```python
from build123d import *

# Parameters (mm, degrees)
SKETCH1_W           = 304.8
SKETCH1_H           = 101.6
BOSS_EXTRUDE1_DEPTH = 6.35
SKETCH2_R           = 12.7
BOSS_EXTRUDE3_DEPTH = 5.55625
SKETCH9_R           = 11.1125
CUT_EXTRUDE4_DEPTH  = 4.445
CUT_EXTRUDE5_START  = -5.55625
SKETCH10_R          = 11.1125
CUT_EXTRUDE5_DEPTH  = 5.55625
SKETCH11_R          = 7.9375
CUT_EXTRUDE6_DEPTH  = 310.094403462
SKETCH12_R          = 12.7
CUT_EXTRUDE7_DEPTH  = 310.0695755
SKETCH22_W          = 63.5
SKETCH22_H          = 63.5
BOSS_EXTRUDE7_DEPTH = 12.7
SKETCH25_W          = 50.8
SKETCH25_H          = 50.8
CUT_EXTRUDE11_DEPTH = 15.24
SKETCH18_W          = 40.386
SKETCH18_H          = 20.066
BOSS_EXTRUDE5_DEPTH = 39.878
SKETCH32_R          = 4.7625
CUT_EXTRUDE12_DEPTH = 6.35


with BuildPart() as part:
    # Sketch1 → Boss-Extrude1 (new body)
    with BuildSketch(Plane(origin=(0, 0, 0), x_dir=(1, 0, 0), z_dir=(0, 1, 0))):
        with Locations((-152.4, 0)):
            Rectangle(SKETCH1_W, SKETCH1_H)
    extrude(amount=BOSS_EXTRUDE1_DEPTH)

    # Sketch2 → Boss-Extrude3 (add)
    with BuildSketch(Plane(origin=(0, 6.35, 0), x_dir=(1, 0, 0), z_dir=(0, 1, 0))):
        with Locations(Location((-282.839226834, 0, 0), (0, 0, 90))):
            Circle(SKETCH2_R)
    extrude(amount=BOSS_EXTRUDE3_DEPTH)

    # Sketch9 → Cut-Extrude4 (cut)
    with BuildSketch(Plane(origin=(0, 11.90625, 0), x_dir=(1, 0, 0), z_dir=(0, 1, 0))):
        with Locations(Location((-282.839226834, 0, 0), (0, 0, 270))):
            Circle(SKETCH9_R)
    extrude(amount=-CUT_EXTRUDE4_DEPTH, mode=Mode.SUBTRACT)

    # Sketch10 → Cut-Extrude5 (cut)
    with BuildSketch(Plane(origin=(0, 0, 0), x_dir=(-1, 0, 0), z_dir=(0, -1, 0)).offset(CUT_EXTRUDE5_START)):
        with Locations(Location((282.839226834, 0, 0), (0, 0, 270))):
            Circle(SKETCH10_R)
    extrude(amount=CUT_EXTRUDE5_DEPTH, mode=Mode.SUBTRACT)

    # Sketch11 → Cut-Extrude6 (cut, through all)
    with BuildSketch(Plane(origin=(0, 7.46125, 0), x_dir=(1, 0, 0), z_dir=(0, 1, 0))):
        with Locations(Location((-282.839226834, 0, 0), (0, 0, 270))):
            Circle(SKETCH11_R)
    extrude(amount=-CUT_EXTRUDE6_DEPTH, mode=Mode.SUBTRACT)

    # Sketch12 → Cut-Extrude7 (cut, through all)
    with BuildSketch(Plane(origin=(0, 6.35, 0), x_dir=(1, 0, 0), z_dir=(0, 1, 0))):
        with Locations(Location((-134.666203771, 0, 0), (0, 0, 270))):
            Circle(SKETCH12_R)
    extrude(amount=-CUT_EXTRUDE7_DEPTH, mode=Mode.SUBTRACT)

    # Sketch22 → Boss-Extrude7 (add)
    with BuildSketch(Plane(origin=(0, 6.35, 0), x_dir=(1, 0, 0), z_dir=(0, 1, 0))):
        with Locations((-134.666203771, 0)):
            Rectangle(SKETCH22_W, SKETCH22_H)
    extrude(amount=BOSS_EXTRUDE7_DEPTH)

    # Sketch25 → Cut-Extrude11 (cut)
    with BuildSketch(Plane(origin=(0, 19.05, 0), x_dir=(1, 0, 0), z_dir=(0, 1, 0))):
        with Locations((-134.666203771, 0)):
            Rectangle(SKETCH25_W, SKETCH25_H)
    extrude(amount=-CUT_EXTRUDE11_DEPTH, mode=Mode.SUBTRACT)

    # Sketch18 → Boss-Extrude5 (add)
    with BuildSketch(Plane(origin=(0, 6.35, 0), x_dir=(1, 0, 0), z_dir=(0, 1, 0))):
        with Locations((-206.419013169, 0)):
            Rectangle(SKETCH18_W, SKETCH18_H)
    extrude(amount=BOSS_EXTRUDE5_DEPTH)

    # Sketch32 → Cut-Extrude12 (cut)
    with BuildSketch(Plane(origin=(0, 6.35, 0), x_dir=(1, 0, 0), z_dir=(0, 1, 0))):
        with Locations(Location((-59.544913048, -40.64, 0), (0, 0, 270))):
            Circle(SKETCH32_R)
        with Locations(Location((-73.514913048, -40.64, 0), (0, 0, 270))):
            Circle(SKETCH32_R)
        with Locations(Location((-59.544913048, 40.64, 0), (0, 0, 270))):
            Circle(SKETCH32_R)
        with Locations(Location((-73.514913048, 40.64, 0), (0, 0, 270))):
            Circle(SKETCH32_R)
    extrude(amount=-CUT_EXTRUDE12_DEPTH, mode=Mode.SUBTRACT)


solid = part.part
```
Input: part model. Units: mm. Frame: model coordinates. A direction names the side the tool comes from. Round coordinates to 2 decimals unless told otherwise and drop trailing zeros. Loops run counter-clockwise (first coordinate to the right, second up) from the corner with the lowest first, then second, coordinate; pieces in that order, holes last. Notation, with made-up numbers: (-18.5, 16) - (-11.5, 16) arc R16 cw to (-11.5, 23) - close; hole circle Ø1 at (0.25, 75). An arc over 180 degrees is marked (long way). One line per item, written item: value. Start each with the question number.
(1) Section B-B, the plane x = -277.5. Return loops of the section in (y, z).
(2) Ray query, line 1 (X direction, y = 3, z = 40.64); line 2 (X direction, y = 1, z = 0); line 3 (X direction, y = 11.5, z = -21). Return the intervals inside material, ascending. Write a range as [from, to].
(3) Contact query for flat-ended pins moving along their axis: P1, Ø14, axis at y = 15, z = -7.5, coming from the +X side; P2, Ø4.5, axis at y = 9, z = 0, coming from the -X side; P3, Ø13.5, axis at x = -282.84, z = 0, coming from the +Y side; P4, Ø10, axis at x = -134, y = 13, coming from the +Z side. Output: stop coordinate, or through.
(4) Draft query along X for faces 5 (the flat face through (-271.6, 11.906, -0.9)), 6 (the cylindrical face through (-271.99, 2.82, -2.41)), 7 (the flat face through (0, 3, 1)). Return one class per face: +X half, -X half, draft (parallel to the pull), parting line (faces both ways), or undercut.
(5) Section A-A, the plane z = -40.64. Return loops of the section in (x, y).
(6) Section D-D, the plane y = 25.5. Return loops of the section in (x, z).
(7) Section C-C, the plane z = -21. Return loops of the section in (x, y).
(8) Access query for faces 1 (the flat face through (-186.226, 26, 0)), 2 (the flat face through (-102.916, 13, 0)), 3 (the flat face through (-285, 5.556, -8)), 4 (the flat face through (-280, 7.461, -8)). Directions: +Z, -Z, +X, -X, +Y, -Y. A direction counts if a zero-diameter tool reaches every point of the face in a straight line with its end or side. Return the directions, or none.
Results below:
1. outline: (0, -50.8) - (6.35, -50.8) - (6.35, -11.52) - (11.91, -11.52) - (11.91, -9.75) - (7.46, -9.75) - (7.46, -5.87) - (5.56, -5.87) - (5.56, -9.75) - (0, -9.75) - close; (0, 9.75) - (5.56, 9.75) - (5.56, 5.87) - (7.46, 5.87) - (7.46, 9.75) - (11.91, 9.75) - (11.91, 11.52) - (6.35, 11.52) - (6.35, 50.8) - (0, 50.8) - close
2. line 1: [-304.8, -78.28], [-68.75, -64.31], [-54.78, 0]
2. line 2: [-304.8, -293.95], [-271.73, -147.37], [-121.97, 0]
2. line 3: [-166.42, -160.07], [-109.27, -102.92]
3. P1: x = -102.92
3. P2: x = -295.54
3. P3: through
3. P4: z = 31.75
4. face 5: draft
4. face 6: undercut
4. face 7: +X half
5. outline: (-304.8, 0) - (-78.28, 0) - (-78.28, 6.35) - (-304.8, 6.35) - close; (-68.75, 0) - (-64.31, 0) - (-64.31, 6.35) - (-68.75, 6.35) - close; (-54.78, 0) - (0, 0) - (0, 6.35) - (-54.78, 6.35) - close
6. outline: (-226.61, -10.03) - (-186.23, -10.03) - (-186.23, 10.03) - (-226.61, 10.03) - close
7. outline: (-304.8, 0) - (0, 0) - (0, 6.35) - (-102.92, 6.35) - (-102.92, 19.05) - (-109.27, 19.05) - (-109.27, 3.81) - (-160.07, 3.81) - (-160.07, 19.05) - (-166.42, 19.05) - (-166.42, 6.35) - (-304.8, 6.35) - close
8. face 1: +Z, -Z, +Y
8. face 2: +Z, -Z, +X, +Y
8. face 3: -Y
8. face 4: +Y
